Read the model definition and answer for the solid it produces. Units are mm, in the model's axes. A direction names the side the tool comes from. Round coordinates to 2 decimals unless told otherwise and drop trailing zeros. Write each loop counter-clockwise with the first axis right and the second up, starting at its lowest first coordinate (ties: lowest second). Pieces come first, ordered by that corner, then holes. Notation, with made-up numbers: (-21.75, 77.25) - (36.25, 77.25) arc R16 ccw to (36.25, 97.25) - close; hole circle Ø3 at (14.5, 47). An arc over 180 degrees is marked (long way). One line per item, written item: value. Start each with the question number.
(1) Flat-ended cylindrical pins translate along their axes: pin 1 Ø1.5 at (x, y) = (14.5, 10.5) entering from +Z; pin 2 Ø8 at (y, z) = (7.5, -3.5) entering from +X; pin 3 Ø1.5 at (y, z) = (6, -21.5) entering from +X. Find the tip coordinate at first contact, or state that the pin passes through.
(2) For faces 4 (the face through (3.68, 7.6, -15.39)), 5 (the face through (1, 11, -3)), 6 (the face through (4.33, 7, -1)), determine the directions among +Z, -Z, +X, -X, +Y, -Y from which every point of the face is accessible in a straight line to the end or side of a thin tool.
(3) A cutting plane is placed at A-A, the plane x = 2.75. Determine the outline of the cut face in (y, z), plus the area to 3 significant figures.
(4) A cutting plane is placed at D-D, the plane x = 16.75. Determine the outline of the cut face in (y, z), plus the area to 3 significant figures.
(5) A cutting plane is placed at C-C, the plane y = 3.75. Determine the outline of the cut face in (x, z).
(6) Find the intervals of material crossed by L1, parallel to Z at x = 4.75, y = 8.25; L2, parallel to Z at x = 4.5, y = 9.75; L3, parallel to X at y = 10.5, z = -15.5, in increasing order.
(7) The mould has two halves that part along Z. Classify faces 1 (the face through (9, 0, -13)), 2 (the face through (1, 13, -3.2)), 3 (the face through (2.75, 7.4, -4.76)): +Z half, -Z half, draft (parallel to the pull), parting line (faces both ways), or undercut.
(8) A cutting plane is placed at B-B, the plane z = -19. Determine the outline of the cut face in (x, y).
Autodesk Inventor part; units mm, degrees
ref_plane "YZ Plane" through (0, 0, 0) normal (1, 0, 0) x (0, 1, 0)
ref_plane "XZ Plane" through (0, 0, 0) normal (0, 1, 0) x (-1, 0, 0)
ref_plane "XY Plane" through (0, 0, 0) normal (0, 0, 1) x (1, 0, 0)
sketch "Sketch22" plane through (0, 0, 0) normal (0, 1, 0) x (-1, 0, 0)
  line L0 (0, 0) -> (-4.3301, 0)
  line L1 (-4.3301, 0) -> (-4.3301, -2.5)
  line L2 (-4.3301, -2.5) -> (-18.3309, -26.75)
  line L3 (-18.3309, -26.75) -> (-16.1658, -28)
  line L4 (-16.1658, -28) -> (0, 0)
  dimension "d180" = 60
  dimension "d182" = 2.5
  dimension "d184" = 2.5
  dimension "d185" = 28
extrude "Extrusion22" add sketch "Sketch22" along normal blind 15
sketch "Sketch23" plane through (0, 15, 0) normal (0, 1, 0) x (1, 0, 0)
  line L0 (16.1658, 28) -> (0, 0)
  arc A0 (6.7017, 19.6077) -> (6.1658, 10.6795) centre (8.6658, 15.0096) ccw
  arc A1 (7.7634, 21.4467) -> (5.4158, 9.3805) centre (8.6658, 15.0096) ccw
  line L1 (18.3309, 26.75) -> (16.1658, 28)
  line L2 (6.7017, 19.6077) -> (7.7634, 21.4467)
  dimension "d188" = 10
  dimension "d189" = 1.5
  dimension "d190" = 15
  dimension "d191" = 4
extrude "Extrusion23" add sketch "Sketch23" against normal blind 15
sketch "Sketch24" plane through (0, 15, 0) normal (0, 1, 0) x (1, 0, 0)
  line L0 (4.3301, 0) -> (4.3301, 2.5)
  line L1 (4.3301, 2.2) -> (-0.1525, 2.2)
  line L2 (0, 0) -> (4.3301, 0)
  line L3 (-0.1525, 2.2) -> (-0.1525, 3.2)
  line L4 (-0.1525, 3.2) -> (1.8475, 3.2)
  line L5 (1.8475, 3.2) -> (1.2702, 2.2)
  line L6 (5.4158, 9.3805) -> (0, 0)
  dimension "d194" = 2.2
  dimension "d195" = 2
  dimension "d196" = 1
extrude "Extrusion24" add sketch "Sketch24" against normal blind 4 contours L1 L3 L4 L5
chamfer "Chamfer6" distance 2 angle 45 2 edges at (17.2483, 15, -27.375) (17.2483, 0, -27.375)
properties part number "part_v3-4_3"
Here are the results:
1. pin 1: z = -18.82
1. pin 2: x = 7.22
1. pin 3: x = 15.73
2. face 4: +Y, -Y
2. face 5: -Z, -X, -Y
2. face 6: +Z, +X, +Y, -Y
3. outline: (0, -17.7) - (15, -17.7) - (15, -12.32) - (0, -12.32) - close; (0, -4.76) - (15, -4.76) - (15, 0) - (0, 0) - close
3. area: 152 mm²
4. outline: (0, -25.35) - (2, -27.66) - (13, -27.66) - (15, -25.35) - (15, -24.01) - (0, -24.01) - close
4. area: 50.1 mm²
5. outline: (0, 0) - (5.42, -9.38) arc R6.5 ccw to (7.76, -21.45) - (6.7, -19.61) arc R5 cw to (6.17, -10.68) - (16.17, -28) - (18.33, -26.75) - (4.33, -2.5) - (4.33, 0) - close
6. L1: -20.2 to -18.12, -11.9 to -9.82, -8.23 to -3.23
6. L2: -20 to -17.77, -12.24 to -10.02, -7.79 to -2.79
6. L3: 2.18 to 3.69, 8.95 to 11.84
7. face 1: draft
7. face 2: -Z half
7. face 3: undercut
8. outline: (3.53, 0) - (5.65, 0) - (5.65, 15) - (3.53, 15) - close; (10.97, 0) - (13.86, 0) - (13.86, 15) - (10.97, 15) - close
